Check sheet for the modelled part. Datum: model origin and axes. Units: mm. A direction names the side the tool comes from. Round coordinates to 2 decimals unless told otherwise and drop trailing zeros. Write each loop counter-clockwise with the first axis right and the second up, starting at its lowest first coordinate (ties: lowest second). Pieces come first, ordered by that corner, then holes.
Item 1: Section check A-A, the plane z = 62. Record the cut outline in (x, y), plus the area to 3 significant figures.
Item 2: Release check for a two-part mould opening along Y. For faces 3 (the cylindrical face through (54.787, 9.48, 73.902)), 4 (the flat face through (48, 12, 50.74)), 5 (the flat face through (48, 12.998, 65)), 6 (the cylindrical face through (46.008, 12.247, 64.644)) record: pulls with the +Y half, pulls with the -Y half, needs draft (parallel to the pull), parting line crosses it, or undercut.
Item 3: Material ranges on line 1 along Y through (x, z) = (41.5, 57); line 2 along Y through (x, z) = (56, 72.5); line 3 along Z through (x, y) = (40.75, 10.75), recorded low to high.
Item 4: Section check B-B, the plane y = -4. Record the cut outline in (x, z), plus the area to 3 significant figures.
Item 5: Section check D-D, the plane x = 51.5. Record the cut outline in (y, z).
Item 6: Set-up check for faces 1 (the cylindrical face through (54.774, 9.703, 55.627)), 2 (the cylindrical face through (55.91, 0.304, 74.004)): record each of +Z, -Z, +X, -X, +Y, -Y from which the full face is reachable in a straight line by a thin tool's end or side.
Item 7: Depth check by flat-ended pin: pin 1 (6 mm diameter, centred on x = 43.5, z = 53, fed in from -Y); pin 2 (13 mm diameter, centred on y = 4, z = 69, fed in from -X); pin 3 (6.5 mm diameter, centred on y = -0.5, z = 64.74, fed in from +X). Enter the tip coordinate at first touch or a pass-through.
Item 8: Section check C-C, the plane y = 0.5. Record the cut outline in (x, z), plus the area to 3 significant figures.
Autodesk Inventor part; units mm, degrees
ref_plane "YZ Plane" through (0, 0, 0) normal (1, 0, 0) x (0, 1, 0)
ref_plane "XZ Plane" through (0, 0, 0) normal (0, 1, 0) x (-1, 0, 0)
ref_plane "XY Plane" through (0, 0, 0) normal (0, 0, 1) x (1, 0, 0)
ref_plane "РабПлоскость1" through (57.3886, 15.9976, 24.7396) normal (1, 0, 0) x (0, 1, 0)
sketch "Эскиз1" plane through (57.3886, 15.9976, 24.7396) normal (1, 0, 0) x (0, 1, 0)
  circle A0 centre (-16.5, 48) radius 1.5
  circle A1 centre (-16.5, 31) radius 1.5
  circle A2 centre (-16.5, 40) radius 4
  line L0 (-3, 26) -> (-3, 54)
  circle A3 centre (-16.5, 40) radius 12.75
  line L1 (-3, 54) -> (-3, 26)
  line L2 (-3, 27.25) -> (-3, 52.75)
  line L3 (-3, 26) -> (-29.25, 26)
  line L4 (-29.25, 26) -> (-29.25, 54)
  line L5 (-29.25, 54) -> (-3, 54)
  line L6 (-3, 54) -> (-3, 26)
  line L7 (-5.5313, 46.5) -> (-5.5313, 54)
  line L8 (-3, 54) -> (-3, 26)
  line L9 (-5.5313, 26) -> (-5.5313, 33.5)
  point P0 (-15.9976, -24.7396)
  point P1 (-3, 26)
  dimension "d15" = 25.5
extrude "Выдавливание1" add sketch "Эскиз1" against normal blind 3 contours A3
extrude "Выдавливание2" add sketch "Эскиз1" against normal blind 20 contours L3 L9 A3 L7 L5 L0
fillet "Сопряжение1" radius 2 1 edges at (55.8886, 10.4663, 58.2396)
fillet "Сопряжение2" radius 2 1 edges at (55.8886, 10.4663, 71.2396)
sketch "Эскиз2" plane through (57.3886, 12.9976, 78.7396) normal (0, 1, 0) x (1, 0, 0)
  point P0 (-57.3886, 78.7396)
sketch "Эскиз4" plane through (57.3886, 12.9976, 78.7396) normal (0, 1, 0) x (1, 0, 0)
  circle A0 centre (-6, 24) radius 1.5
  circle A1 centre (-6, 24) radius 3.5
  circle A2 centre (-6, 4) radius 1.5
  circle A3 centre (-6, 4) radius 3.5
  circle A4 centre (-16, 4) radius 1.5
  circle A5 centre (-16, 4) radius 3.5
  circle A6 centre (-16, 24) radius 1.5
  circle A7 centre (-16, 24) radius 3.5
  point P0 (-57.3886, 78.7396)
  dimension "d33" = 7
  dimension "d34" = 7
  dimension "d35" = 7
  dimension "d36" = 7
extrude "Выдавливание5" cut sketch "Эскиз4" against normal blind 2 from surface at -2.5313
properties part number "крепёж_мотора_прототип"
Values found:
1. outline: (37.39, 11.95) - (54.39, 11.95) - (54.39, 2.41) - (57.39, 2.41) - (57.39, 13) - (37.39, 13) - close; (54.39, -12.95) - (57.39, -12.95) - (57.39, -3.42) - (54.39, -3.42) - close
1. area: 78.2 mm2
2. face 3: undercut
2. face 4: needs draft
2. face 5: pulls with the +Y half
2. face 6: pulls with the -Y half
3. line 1: y = 10.47 to 13
3. line 2: y = -10.62 to -1.98, 0.98 to 13
3. line 3: z = 50.74 to 58.74, 70.74 to 78.74
4. outline: (54.39, 52.48) - (57.39, 52.48) - (57.39, 62.8) - (54.39, 62.8) - close; (54.39, 66.68) - (57.39, 66.68) - (57.39, 77) - (54.39, 77) - close
4. area: 61.9 mm2
5. outline: (10.47, 50.74) - (13, 50.74) - (13, 78.74) - (10.47, 78.74) - (10.47, 71.24) arc R12.75 cw to (10.47, 58.24) - close
6. face 1: -X
6. face 2: +X, -X
7. pin 1: stops at y = 10.47
7. pin 2: stops at x = 54.39
7. pin 3: passes through
8. outline: (54.39, 52.03) - (57.39, 52.03) - (57.39, 54.62) - (54.39, 54.62) - close; (54.39, 56.86) - (57.39, 56.86) - (57.39, 60.87) - (54.39, 60.87) - close; (54.39, 68.61) - (57.39, 68.61) - (57.39, 71.62) - (54.39, 71.62) - close; (54.39, 73.86) - (57.39, 73.86) - (57.39, 77.45) - (54.39, 77.45) - close
8. area: 39.6 mm2
